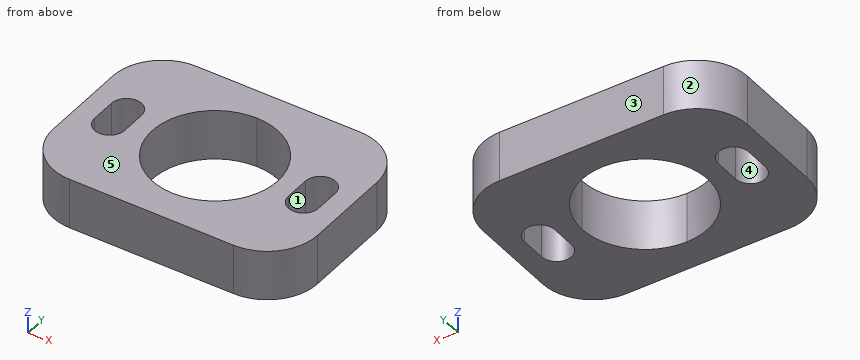
```python
from build123d import *

# Parameters (mm, degrees)
BOSS_EXTRUDE1_DEPTH = 6.35
FILLET1_R           = 6.35


with BuildPart() as part:
    # Sketch1 → Boss-Extrude1 (new body)
    # profile 1 of 6: a face of its own
    with BuildSketch(Plane.XY.offset(-95.039403682)):
        with BuildLine():
            ThreePointArc((15.304322218, 15.940467802), (6.541322218, 24.703467802), (15.304322218, 33.466467802))
            Line((15.304322218, 33.466467802), (15.304322218, 36.641467802))
            Line((15.304322218, 36.641467802), (-1.408877782, 36.641467802))
            Line((-1.408877782, 36.641467802), (-1.408877782, 12.765467802))
            Line((-1.408877782, 12.765467802), (15.304322218, 12.765467802))
            Line((15.304322218, 12.765467802), (15.304322218, 15.940467802))
        make_face()
        with BuildLine():
            Line((1.143822218, 23.115967802), (1.143822218, 26.290967802))
            ThreePointArc((1.143822218, 26.290967802), (3.048822218, 28.195967802), (4.953822218, 26.290967802))
            Line((4.953822218, 26.290967802), (4.953822218, 23.115967802))
            ThreePointArc((4.953822218, 23.115967802), (3.048822218, 21.210967802), (1.143822218, 23.115967802))
        make_face(mode=Mode.SUBTRACT)
    # profile 2 of 6: a face of its own
    with BuildSketch(Plane.XY.offset(-95.039403682)):
        with BuildLine():
            Line((15.304322218, 36.641467802), (15.304322218, 33.466467802))
            ThreePointArc((15.304322218, 33.466467802), (21.500698942, 30.899844525), (24.067322218, 24.703467802))
            ThreePointArc((24.067322218, 24.703467802), (21.500698942, 18.507091078), (15.304322218, 15.940467802))
            Line((15.304322218, 15.940467802), (15.304322218, 12.765467802))
            Line((15.304322218, 12.765467802), (32.017522218, 12.765467802))
            Line((32.017522218, 12.765467802), (32.017522218, 36.641467802))
            Line((32.017522218, 36.641467802), (15.304322218, 36.641467802))
        make_face()
        with BuildLine():
            Line((25.654822218, 23.115967802), (25.654822218, 26.290967802))
            ThreePointArc((25.654822218, 26.290967802), (27.559822218, 28.195967802), (29.464822218, 26.290967802))
            Line((29.464822218, 26.290967802), (29.464822218, 23.115967802))
            ThreePointArc((29.464822218, 23.115967802), (27.559822218, 21.210967802), (25.654822218, 23.115967802))
        make_face(mode=Mode.SUBTRACT)
    # profile 3 of 6: a face of its own
    with BuildSketch(Plane.XY.offset(-95.039403682)):
        with BuildLine():
            ThreePointArc((15.304322218, 16.765967802), (7.366822218, 24.703467802), (15.304322218, 32.640967802))
            Line((15.304322218, 32.640967802), (15.304322218, 33.466467802))
            ThreePointArc((15.304322218, 33.466467802), (6.541322218, 24.703467802), (15.304322218, 15.940467802))
            Line((15.304322218, 15.940467802), (15.304322218, 16.765967802))
        make_face()
    # profile 4 of 6: a face of its own
    with BuildSketch(Plane.XY.offset(-95.039403682)):
        with BuildLine():
            Line((15.304322218, 33.466467802), (15.304322218, 32.640967802))
            ThreePointArc((15.304322218, 32.640967802), (20.916982294, 30.316127877), (23.241822218, 24.703467802))
            ThreePointArc((23.241822218, 24.703467802), (20.916982294, 19.090807726), (15.304322218, 16.765967802))
            Line((15.304322218, 16.765967802), (15.304322218, 15.940467802))
            ThreePointArc((15.304322218, 15.940467802), (21.500698942, 18.507091078), (24.067322218, 24.703467802))
            ThreePointArc((24.067322218, 24.703467802), (21.500698942, 30.899844525), (15.304322218, 33.466467802))
        make_face()
    # profile 5 of 6: a face of its own
    with BuildSketch(Plane.XY.offset(-95.039403682)):
        with BuildLine():
            ThreePointArc((15.304322218, 16.765967802), (7.366822218, 24.703467802), (15.304322218, 32.640967802))
            Line((15.304322218, 32.640967802), (15.304322218, 33.466467802))
            ThreePointArc((15.304322218, 33.466467802), (6.541322218, 24.703467802), (15.304322218, 15.940467802))
            Line((15.304322218, 15.940467802), (15.304322218, 16.765967802))
        make_face()
    # profile 6 of 6: a face of its own
    with BuildSketch(Plane.XY.offset(-95.039403682)):
        with BuildLine():
            Line((15.304322218, 33.466467802), (15.304322218, 32.640967802))
            ThreePointArc((15.304322218, 32.640967802), (20.916982294, 30.316127877), (23.241822218, 24.703467802))
            ThreePointArc((23.241822218, 24.703467802), (20.916982294, 19.090807726), (15.304322218, 16.765967802))
            Line((15.304322218, 16.765967802), (15.304322218, 15.940467802))
            ThreePointArc((15.304322218, 15.940467802), (21.500698942, 18.507091078), (24.067322218, 24.703467802))
            ThreePointArc((24.067322218, 24.703467802), (21.500698942, 30.899844525), (15.304322218, 33.466467802))
        make_face()
    extrude(amount=BOSS_EXTRUDE1_DEPTH)

    # Fillet1
    fillet1_edges = [part.edges().sort_by_distance(p)[0] for p in [
        (32.017522218, 12.765467802, -91.864403682),
        (-1.408877782, 12.765467802, -91.864403682),
        (-1.408877782, 36.641467802, -91.864403682),
        (32.017522218, 36.641467802, -91.864403682),
    ]]
    fillet(fillet1_edges, radius=FILLET1_R)


solid = part.part
```
Build history of the part. All positions in model axes, mm. Face numbers are marked on the shaded views. A direction names the side the tool comes from. Give positions to 0.01 mm unless a question says otherwise; leave off trailing zeros. Order: outer loops, then holes, each group sorted by start corner. A loop starts at its lowest first (then second) coordinate and runs counter-clockwise, first axis right, second up. Notation, with made-up numbers: M -8.75,13.25 L 29.25,13.25 A10 ccw 29.25,20.25 Z; hole C 37.5,35.25 d4. An arc over 180 degrees is marked long. Return JSON: item names as keys, results as strings.
Q1. Band-saw the part on D-D (y = 31.25). Give the cut face in (x, z), then the cut area to 3 significant figures.
Answer list:
{"outline": "M -1.34,-95.04 L 10.82,-95.04 L 10.82,-88.69 L -1.34,-88.69 Z; M 19.79,-95.04 L 31.94,-95.04 L 31.94,-88.69 L 19.79,-88.69 Z", "area": "154 mm^2"}
Q2. Band-saw the part on A-A (z = -89.75). Count the separate pieces of the cut face and the enclosed holes in it, then the cut area to 3 significant figures.
Answer list:
{"separate pieces": "1", "enclosed holes": "3", "area": "519 mm^2"}
Q3. Wall check: probe 1 along X at (y, z) = (26, -94.5); probe 2 along X at (y, z) = (22.75, -91.25); probe 3 along Y at (x, z) = (8.5, -90). Give the ranges that are in metal, low to high. Write a range as from..to.
Answer list:
{"probe 1": "x = -1.41..1.14, 4.95..7.47, 23.14..25.65, 29.46..32.02", "probe 2": "x = -1.41..1.18, 4.92..7.61, 23..25.69, 29.43..32.02", "probe 3": "y = 12.77..20.62, 28.79..36.64"}
Q4. 3-axis set-ups, long thin cutter, end or side, ignore diameter. For the marked faces 4 and 5: which of +Z, -Z, +X, -X, +Y, -Y reach the whole face in a straight line?
Answer list:
{"face 4": "+Z, -Z", "face 5": "+Z, +X, -X, +Y, -Y"}
Q5. Band-saw the part on C-C (y = 22.25). Give the cut face in (x, z), then the cut area to 3 significant figures.
Answer list:
{"outline": "M -1.41,-95.04 L 1.35,-95.04 L 1.35,-88.69 L -1.41,-88.69 Z; M 4.75,-95.04 L 7.76,-95.04 L 7.76,-88.69 L 4.75,-88.69 Z; M 22.85,-95.04 L 25.86,-95.04 L 25.86,-88.69 L 22.85,-88.69 Z; M 29.26,-95.04 L 32.02,-95.04 L 32.02,-88.69 L 29.26,-88.69 Z", "area": "73.3 mm^2"}
Q6. Two-plate mould, pull along X, no slides. Class the marked faces 1, 2 and 3: pulls with the +X half, pulls with the -X half, needs draft (parallel to the pull), parting line crosses it, or undercut.
Answer list:
{"face 1": "undercut", "face 2": "pulls with the -X half", "face 3": "needs draft"}
Q7. Band-saw the part on B-B (x = 14). Give the cut face in (y, z).
Answer list:
{"outline": "M 12.77,-95.04 L 16.87,-95.04 L 16.87,-88.69 L 12.77,-88.69 Z; M 32.53,-95.04 L 36.64,-95.04 L 36.64,-88.69 L 32.53,-88.69 Z"}
